from build123d import *


with BuildPart() as part:
    # Pin: sweep along a path in Sketch1
    with BuildLine(Plane.XY) as pin_path:
        Line((0.025, -6.223), (0.025, -1.681188568))
        ThreePointArc((0.025, -1.681188568), (0.153227812, -1.069309495), (0.516333333, -0.560396189))
        ThreePointArc((0.516333333, -0.560396189), (0, 0.762), (-0.516333333, -0.560396189))
        ThreePointArc((-0.516333333, -0.560396189), (-0.153227812, -1.069309495), (-0.025, -1.681188568))
        Line((-0.025, -1.681188568), (-0.025, -6.2357))
        ThreePointArc((-0.025, -6.2357), (-0.808992041, -7.409027006), (-2.193025612, -7.133725612))
        Line((-2.193025612, -7.133725612), (-3.719669153, -5.607082072))
    # Sketch2 → Pin (sweep)
    with BuildSketch(Plane(origin=(0.025, -6.223, 0), x_dir=(1, 0, 0), z_dir=(0, -1, 0))):
        with BuildLine():
            Line((0, 0.8001), (0, -0.8001))
            ThreePointArc((0, -0.8001), (0.8001, 0), (0, 0.8001))
        make_face()
    sweep(path=pin_path.line)

    # Sweep1: sweep along a path in Sketch3
    with BuildLine(Plane.XY) as sweep1_path:
        Line((3.54006403, -5.773987194), (2.193025612, -7.121025612))
        ThreePointArc((2.193025612, -7.121025612), (0.808992041, -7.396327006), (0.025, -6.223))
    # Sketch4 → Sweep1 (sweep)
    with BuildSketch(Plane.XZ.offset(6.223)):
        with BuildLine():
            Line((0.025, 0.8001), (0.025, -0.8001))
            ThreePointArc((0.025, -0.8001), (0.8251, 0), (0.025, 0.8001))
        make_face()
    sweep(path=sweep1_path.line)


solid = part.part
Input: part model. Units: mm. Frame: model coordinates. A direction names the side the tool comes from. Coordinates: 2 decimals unless noted, no trailing zeros. Loops run counter-clockwise (first coordinate to the right, second up) from the corner with the lowest first, then second, coordinate; pieces in that order, holes last. Notation, with made-up numbers: (-16, 25.25) - (41, 25.25) arc R21 ccw to (41, 31.25) - close; hole circle Ø2 at (40.25, -3.5). An arc over 180 degrees is marked (long way). Answer in a Markdown table with one row per item. Add a question column.
Item 1: Mould query, pull axis Y, two halves, no side actions, for faces 4 (the cylindrical face through (-0.79, -7.4, -0.01)), 5 (the cylindrical face through (-2.401, -5.794, 0.018)), 6 (the cylindrical face through (-0.157, -1.061, -0.011)). Classes: released by +Y, released by -Y, zero draft, split by the parting line, or undercut.
Item 2: Section query A-A on y = -4.5. Return the cut outline in (x, z) (3 decimals).
Item 3: Line query: line 1 along X through (y, z) = (0, 0); line 2 along X through (y, z) = (-1.25, 0.25); line 3 along Y through (x, z) = (1, -0.3). Output: solid intervals per line, ascending. Write a range as [from, to].
Item 4: Access query for faces 1 (the cylindrical face through (0.825, -3.92, 0.018)), 2 (the cylindrical face through (2.291, -5.891, 0.018)), 3 (the cylindrical face through (0.15, -1.08, -0.01)). Directions: +Z, -Z, +X, -X, +Y, -Y. A direction counts if a zero-diameter tool reaches every point of the face in a straight line with its end or side. Return the directions, or none.
Item 5: Contact query for flat-ended pins moving along their axis: P1, Ø2, axis at x = 3, y = -2, coming from the -Z side; P2, Ø0.8, axis at y = -4.5, z = 0, coming from the +X side; P3, Ø0.8, axis at y = -3, z = 0, coming from the -X side. Output: stop coordinate, or through.
Recorded:
| question | item | result |
|---|---|---|
| 1 | face 4 | released by -Y |
| 1 | face 5 | released by +Y |
| 1 | face 6 | undercut |
| 2 | outline | (-0.025, -0.8) - (-0.025, 0.8) arc R0.8 ccw to start; (0.025, -0.8) arc R0.8 ccw to (0.025, 0.8) - close |
| 3 | line 1 | [-1.56, -0.76], [0.76, 1.56] |
| 3 | line 2 | [-0.92, -0.09], [0.09, 0.92] |
| 3 | line 3 | [-7.46, -6.66], [-1.12, 1.12] |
| 4 | face 1 | none |
| 4 | face 2 | +Y |
| 4 | face 3 | +Z, -Z |
| 5 | P1 | through |
| 5 | P2 | x = 0.83 |
| 5 | P3 | x = -0.83 |
